Part model, mm, in its own coordinate system. Face numbers are marked on the shaded views. Coordinates: 2 decimals unless noted, no trailing zeros. Write each loop counter-clockwise with the first axis right and the second up, starting at its lowest first coordinate (ties: lowest second). Pieces come first, ordered by that corner, then holes. Notation, with made-up numbers: (48, 56) -> (60, 56) arc R29 ccw to (60, 93) -> close; hole circle Ø11 at (1, 8). An arc over 180 degrees is marked (long way). Write item = value, one per line. Start each with the question number.
Q1. Band-saw the part on D-D, the plane x = 2.5. List the corners of the cut face in (y, z).
Q2. Band-saw the part on B-B, the plane z = 1.75. Give the number of separate pieces and of enclosed holes in the cut face, plus the area to 3 significant figures.
Q3. Pull direction Y, two halves, no side cores. Call the marked faces 1, 2 and 3: released by +Y, released by -Y, zero draft, split by the parting line, or undercut.
Q4. Probe line 1 (X direction, y = -6, z = 3.3); line 2 (Y direction, x = 0, z = 3.65) (3 decimals); line 3 (Y direction, x = -8, z = 0.75). List the from-to ranges inside material, lowest first.
Q5. Band-saw the part on C-C, the plane y = -5.5. List the corners of the cut face in (x, z).
Q6. Band-saw the part on A-A, the plane x = -1.5. List the corners of the cut face in (y, z).
Q7. Pin check, flat tip, straight feed: P1, Ø3, axis at x = -11.54, y = -5.99, coming from the -Z side. Stop position of the tip, or through.
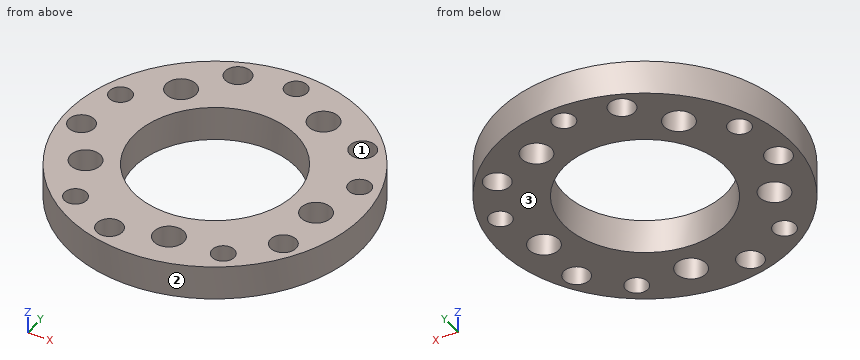
from build123d import *

# Parameters (mm, degrees)
SKETCH_1_R      = 17.25
SKETCH_1_R_2    = 9.485
SKETCH_1_R_3    = 1.3
SKETCH_1_R_4    = 1.5
SKETCH_1_R_5    = 1.75
EXTRUDE_1_DEPTH = 4


with BuildPart() as part:
    # 草图1 → 凸台-拉伸1 (new body)
    with BuildSketch(Plane.XY):
        Circle(SKETCH_1_R)
        Circle(SKETCH_1_R_2, mode=Mode.SUBTRACT)
        with Locations((8.264326198, -12.518023506)):
            Circle(SKETCH_1_R_3, mode=Mode.SUBTRACT)
        with Locations((-9.351530584, -11.728123283)):
            Circle(SKETCH_1_R_3, mode=Mode.SUBTRACT)
        with Locations((-14.043889946, 5.269644693)):
            Circle(SKETCH_1_R_3, mode=Mode.SUBTRACT)
        with Locations((0.671929263, 14.984942812)):
            Circle(SKETCH_1_R_3, mode=Mode.SUBTRACT)
        with Locations((14.459165069, 3.991559284)):
            Circle(SKETCH_1_R_3, mode=Mode.SUBTRACT)
        with Locations((11.585591146, 9.527543115)):
            Circle(SKETCH_1_R_4, mode=Mode.SUBTRACT)
        with Locations((12.641376517, -8.074379217)):
            Circle(SKETCH_1_R_4, mode=Mode.SUBTRACT)
        with Locations((-3.772790794, -14.517783909)):
            Circle(SKETCH_1_R_4, mode=Mode.SUBTRACT)
        with Locations((-14.97308946, -0.89810468)):
            Circle(SKETCH_1_R_4, mode=Mode.SUBTRACT)
        with Locations((-5.481087409, 13.962724691)):
            Circle(SKETCH_1_R_4, mode=Mode.SUBTRACT)
        with Locations((5.814261494, 11.627311094)):
            Circle(SKETCH_1_R_5, mode=Mode.SUBTRACT)
        with Locations((12.854935594, -1.936654554)):
            Circle(SKETCH_1_R_5, mode=Mode.SUBTRACT)
        with Locations((2.130525627, -12.824229433)):
            Circle(SKETCH_1_R_5, mode=Mode.SUBTRACT)
        with Locations((-11.538198343, -5.989155115)):
            Circle(SKETCH_1_R_5, mode=Mode.SUBTRACT)
        with Locations((-9.261524372, 9.122728008)):
            Circle(SKETCH_1_R_5, mode=Mode.SUBTRACT)
    extrude(amount=EXTRUDE_1_DEPTH)


solid = part.part
Ans:
q1.outline = (-17.07, 0) -> (-14.53, 0) -> (-14.53, 4) -> (-17.07, 4) -> close; (-11.11, 0) -> (-9.15, 0) -> (-9.15, 4) -> (-11.11, 4) -> close; (9.15, 0) -> (17.07, 0) -> (17.07, 4) -> (9.15, 4) -> close
q2.separate_pieces = 1
q2.enclosed_holes = 16
q2.area = 542 mm2
q3.face_1 = undercut
q3.face_2 = split by the parting line
q3.face_3 = zero draft
q4.line_1 = -16.17 to -13.29, -9.79 to -7.35, 7.35 to 16.17
q4.line_2 = -17.25 to -9.485, 9.485 to 13.872, 16.098 to 17.25
q4.line_3 = -15.28 to -5.1, 5.1 to 7.91, 10.34 to 15.28
q5.outline = (-16.35, 0) -> (-13.22, 0) -> (-13.22, 4) -> (-16.35, 4) -> close; (-9.86, 0) -> (-7.73, 0) -> (-7.73, 4) -> (-9.86, 4) -> close; (7.73, 0) -> (16.35, 0) -> (16.35, 4) -> (7.73, 4) -> close
q6.outline = (-17.18, 0) -> (-9.37, 0) -> (-9.37, 4) -> (-17.18, 4) -> close; (9.37, 0) -> (17.18, 0) -> (17.18, 4) -> (9.37, 4) -> close
q7.P1 = through
